Here's the drawing with two shaded views (mm, measured from the low corner). I have some questions. Round coordinates to 2 decimals unless told otherwise and drop trailing zeros. Write each loop counter-clockwise with the first axis right and the second up, starting at its lowest first coordinate (ties: lowest second). Pieces come first, ordered by that corner, then holes.
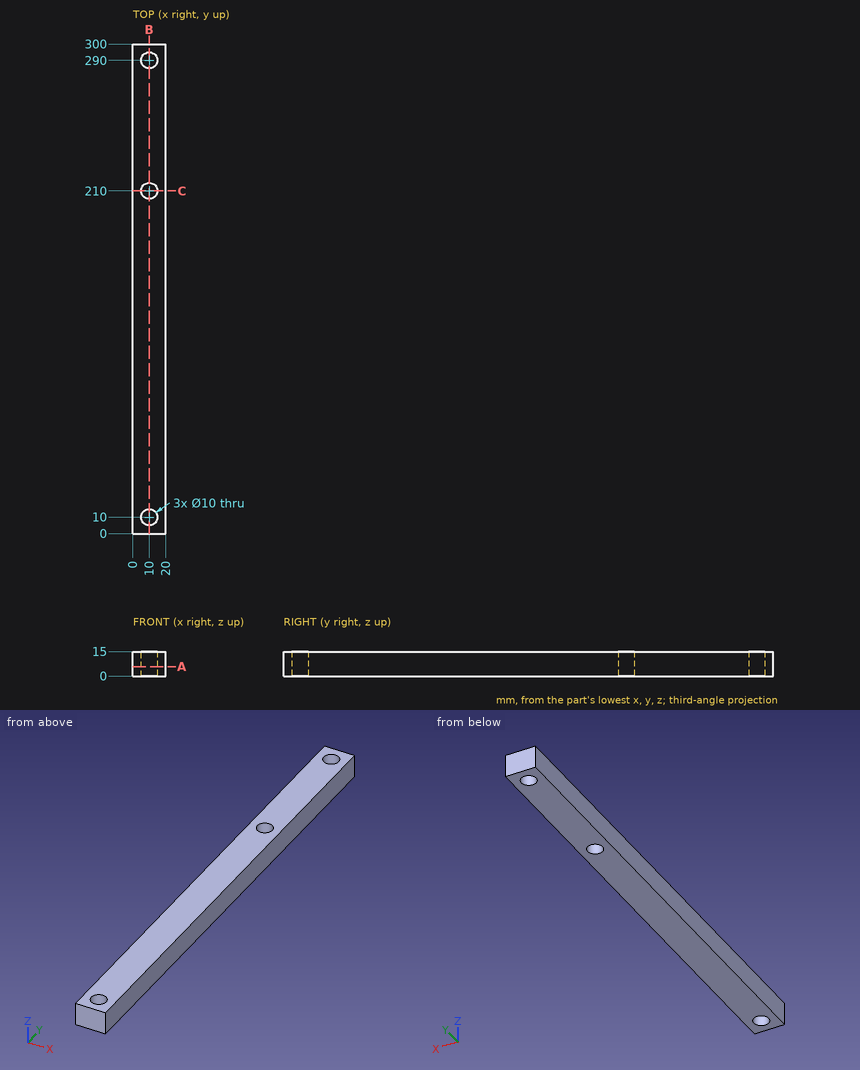
Q1. If I drill on L1, parallel to Y at x = 10, z = 5.25; L2, parallel to X at y = 290, z = 4.25; L3, parallel to Y at x = 7.75, z = 5.25, over which ranges is the centre line in solid material (lowest first)?
Q2. Imagine slicing it at B-B, the plane x = 10. Write out the boundary of the cut face in (y, z).
Q3. Imagine slicing it at A-A, the plane z = 5.75. Write out the boundary of the cut face in (x, y), then the cut area to 3 significant figures.
Q4. Imagine slicing it at C-C, the plane y = 210. Write out the boundary of the cut face in (x, z), then the cut area to 3 significant figures.
Results found:
1. L1: y = 0 to 5, 15 to 205, 215 to 285, 295 to 300
1. L2: x = 0 to 5, 15 to 20
1. L3: y = 0 to 5.53, 14.47 to 205.53, 214.47 to 285.53, 294.47 to 300
2. outline: (0, 0) - (5, 0) - (5, 15) - (0, 15) - close; (15, 0) - (205, 0) - (205, 15) - (15, 15) - close; (215, 0) - (285, 0) - (285, 15) - (215, 15) - close; (295, 0) - (300, 0) - (300, 15) - (295, 15) - close
3. outline: (0, 0) - (20, 0) - (20, 300) - (0, 300) - close; hole circle Ø10 at (10, 10); hole circle Ø10 at (10, 210); hole circle Ø10 at (10, 290)
3. area: 5,760 mm2
4. outline: (0, 0) - (5, 0) - (5, 15) - (0, 15) - close; (15, 0) - (20, 0) - (20, 15) - (15, 15) - close
4. area: 150 mm2
